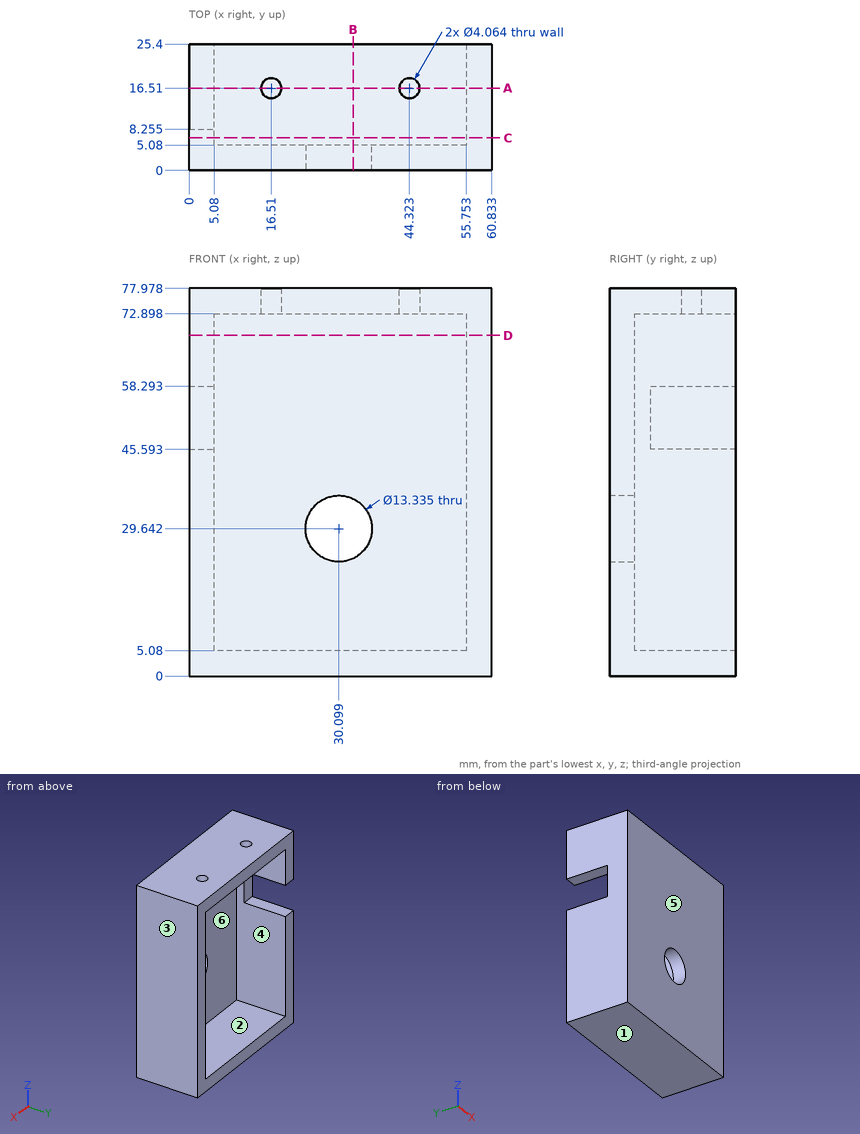
Can you work these out from the drawing? Everything is in mm from the part's minimum corner. A direction names the side the tool comes from. Give positions to 0.01 mm unless a question says otherwise; leave off trailing zeros. Order: outer loops, then holes, each group sorted by start corner. A loop starts at its lowest first (then second) coordinate and runs counter-clockwise, first axis right, second up. Notation, with made-up numbers: M 40,38.25 L 61,38.25 A22 ccw 61,67.25 Z; hole C -26.5,4 d3. An arc over 180 degrees is marked long. Use a Markdown table: item, result. Add a question column.
1. For pin 1 Ø4 at (x, z) = (3, 51) entering from +Y (3 decimals); pin 2 Ø5 at (x, z) = (26.5, 59) entering from +Y, each with a flat end and sliding along its axis, tell me the tip position at first contact or that it passes through.
2. Suppose I cut it at C-C (y = 6.5). List the corners of the cut face in (x, z) for me.
3. I need wall thicknesses on probe 1 along X at (y, z) = (16.51, 75.4) (3 decimals); probe 2 along X at (y, z) = (21.75, 64.5); probe 3 along Z at (x, y) = (21, 6.25). Which ranges of each line are inside material? Lowest first, please. Write a range as from..to.
4. Suppose I cut it at A-A (y = 16.51). List the corners of the cut face in (x, z) for me (3 decimals).
5. If we mould it in two halves opening along X, with no side actions, what happens to the marked faces 3, 4, 5 and 6? For each: +X half, -X half, draft (parallel to the pull), parting line (faces both ways), or undercut.
6. Suppose I cut it at D-D (z = 68.5). List the corners of the cut face in (x, y) for me.
7. On a 3-axis mill with a long thin cutter (end or side, diameter ignored), from which of +Z, -Z, +X, -X, +Y, -Y can I reach the whole of each face in a straight line? I mean the marked faces 1 and 2. Say none if no direction works.
8. Suppose I cut it at B-B (x = 33). List the corners of the cut face in (y, z) for me (1 decimal).
Results list:
| question | item | result |
|---|---|---|
| 1 | pin 1 | stops at y = 8.255 |
| 1 | pin 2 | stops at y = 5.08 |
| 2 | outline | M 0,0 L 60.83,0 L 60.83,77.98 L 0,77.98 Z; hole M 5.08,5.08 L 55.75,5.08 L 55.75,72.9 L 5.08,72.9 Z |
| 3 | probe 1 | x = 0..14.478, 18.542..42.291, 46.355..60.833 |
| 3 | probe 2 | x = 0..5.08, 55.75..60.83 |
| 3 | probe 3 | z = 0..5.08, 72.9..77.98 |
| 4 | outline | M 0,0 L 60.833,0 L 60.833,77.978 L 46.355,77.978 L 46.355,72.898 L 55.753,72.898 L 55.753,5.08 L 5.08,5.08 L 5.08,45.593 L 0,45.593 Z; M 0,58.293 L 5.08,58.293 L 5.08,72.898 L 14.478,72.898 L 14.478,77.978 L 0,77.978 Z; M 18.542,72.898 L 42.291,72.898 L 42.291,77.978 L 18.542,77.978 Z |
| 5 | face 3 | +X half |
| 5 | face 4 | undercut |
| 5 | face 5 | draft |
| 5 | face 6 | undercut |
| 6 | outline | M 0,0 L 60.83,0 L 60.83,25.4 L 55.75,25.4 L 55.75,5.08 L 5.08,5.08 L 5.08,25.4 L 0,25.4 Z |
| 7 | face 1 | -Z, +X, -X, +Y, -Y |
| 7 | face 2 | +Y |
| 8 | outline | M 0,0 L 25.4,0 L 25.4,5.1 L 5.1,5.1 L 5.1,23.6 L 0,23.6 Z; M 0,35.6 L 5.1,35.6 L 5.1,72.9 L 25.4,72.9 L 25.4,78 L 0,78 Z |
